from build123d import *

# Parameters (mm, degrees)
SKETCH1_W           = 58
SKETCH1_H           = 68
SKETCH1_W_2         = 20
SKETCH1_H_2         = 48
BOSS_EXTRUDE1_DEPTH = 3
FILLET2_R           = 5
FILLET3_R           = 5


with BuildPart() as part:
    # Sketch1 → Boss-Extrude1 (new body)
    with BuildSketch(Plane.XY):
        with Locations((29, 34)):
            Rectangle(SKETCH1_W, SKETCH1_H)
        with Locations((15, 34)):
            Rectangle(SKETCH1_W_2, SKETCH1_H_2, mode=Mode.SUBTRACT)
    extrude(amount=BOSS_EXTRUDE1_DEPTH)

    # Fillet2
    fillet2_edges = [part.edges().sort_by_distance(p)[0] for p in [
        (0, 68, 1.5),
        (58, 68, 1.5),
        (58, 0, 1.5),
        (0, 0, 1.5),
    ]]
    fillet(fillet2_edges, radius=FILLET2_R)

    # Fillet3
    fillet3_edges = [part.edges().sort_by_distance(p)[0] for p in [
        (5, 58, 1.5),
        (5, 10, 1.5),
        (25, 10, 1.5),
        (25, 58, 1.5),
    ]]
    fillet(fillet3_edges, radius=FILLET3_R)


solid = part.part
Input: part model. Units: mm. Frame: model coordinates. A direction names the side the tool comes from. Round coordinates to 2 decimals unless told otherwise and drop trailing zeros. Order: outer loops, then holes, each group sorted by start corner. A loop starts at its lowest first (then second) coordinate and runs counter-clockwise, first axis right, second up.
1. Cut plane C-C, the plane y = 32. Output: boundary loops of the cut face in (x, z).
The answers:
outline: (0, 0) - (5, 0) - (5, 3) - (0, 3) - close; (25, 0) - (58, 0) - (58, 3) - (25, 3) - close
2. Material intervals for line 1 (Y direction, x = 19.5, z = 2.25); line 2 (X direction, y = 22.5, z = 1.4); line 3 (Y direction, x = 8, z = 2.1), sorted ascending.
The answers:
line 1: y = 0 to 10, 58 to 68
line 2: x = 0 to 5, 25 to 58
line 3: y = 0 to 10.42, 57.58 to 68
3. Cut plane A-A, the plane x = 6. Output: boundary loops of the cut face in (y, z), then the cut area to 3 significant figures.
The answers:
outline: (0, 0) - (12, 0) - (12, 3) - (0, 3) - close; (56, 0) - (68, 0) - (68, 3) - (56, 3) - close
area: 72.0 mm2
4. Mould query, pull axis X, two halves, no side actions, for faces 3 (the face through (23, 11, 2)), 4 (the face through (35, 34, 3)), 5 (the face through (1, 2, 2)). Classes: released by +X, released by -X, zero draft, split by the parting line, or undercut.
The answers:
face 3: undercut
face 4: zero draft
face 5: released by -X
5. Cut plane B-B, the plane z = 2.55. Output: boundary loops of the cut face in (x, y).
The answers:
outline: (0, 5) arc R5 ccw to (5, 0) - (53, 0) arc R5 ccw to (58, 5) - (58, 63) arc R5 ccw to (53, 68) - (5, 68) arc R5 ccw to (0, 63) - close; hole (5, 15) arc R5 ccw to (10, 10) - (20, 10) arc R5 ccw to (25, 15) - (25, 53) arc R5 ccw to (20, 58) - (10, 58) arc R5 ccw to (5, 53) - close
6. Set-up query: faces 1 (the face through (1, 66, 2)), 2 (the face through (7, 11, 2)). Return all of +Z, -Z, +X, -X, +Y, -Y with unobstructed straight access to the full face (end or side cutting, diameter ignored); none if empty.
The answers:
face 1: +Z, -Z, -X, +Y
face 2: +Z, -Z
